Geometry check sheet. Reference: the model listing, model coordinates, mm. Give positions to 0.01 mm unless a question says otherwise; leave off trailing zeros. Loops run counter-clockwise (first coordinate to the right, second up) from the corner with the lowest first, then second, coordinate; pieces in that order, holes last. Notation, with made-up numbers: (-18.5, -0.75) -> (40.5, -0.75) arc R11 cw to (40.5, 7.25) -> close; hole circle Ø2 at (63.5, 82). An arc over 180 degrees is marked (long way). Write item = value, one per line.
```python
from build123d import *

# Parameters (mm, degrees)
F1_DEPTH    = 10.16
F3_D        = 6.35
F4_T1_DEPTH = 76.2


# Not quite as in the source:
# - a fillet or chamfer that OpenCascade refuses, or shapes differently, is made with other operations: its cross-section is extruded or revolved along the edge and cut away or added


with BuildPart() as f1:
    # F0 (on Front) → F1 (new body)
    with BuildSketch(Plane.XZ):
        Polygon((-25.4, 0), (0, 0), (25.4, 0), (25.4, 10.1957246661), (0, 10.1957246661), (-25.4, 10.1957246661), align=None)
    extrude(amount=F1_DEPTH)

    # F3 (through all)
    with Locations(Plane(origin=(0, 0, 0), x_dir=(1, 0, 0), z_dir=(0, 0, -1))):
        with Locations((0.0320593305, 5.0682155415)):
            Hole(F3_D / 2)

    # F4: fillet of radius 5.08 on 4 edges, made by hand

    # F4_s2 → F4_t1 (cut)
    with BuildSketch(Plane.YZ.offset(-38.1)):
        with BuildLine():
            ThreePointArc((-10.16, 5.1157246661), (-8.6721024484, 8.7078271145), (-5.08, 10.1957246661))
            Line((-5.08, 10.1957246661), (-10.16, 10.1957246661))
            Line((-10.16, 10.1957246661), (-10.16, 5.1157246661))
        make_face()
        with BuildLine():
            ThreePointArc((0, 5.1157246661), (-1.4878975516, 8.7078271145), (-5.08, 10.1957246661))
            Line((-5.08, 10.1957246661), (0, 10.1957246661))
            Line((0, 10.1957246661), (0, 5.1157246661))
        make_face()
        with BuildLine():
            ThreePointArc((-5.08, 0), (-8.6721024484, 1.4878975516), (-10.16, 5.08))
            Line((-10.16, 5.08), (-10.16, 0))
            Line((-10.16, 0), (-5.08, 0))
        make_face()
        with BuildLine():
            ThreePointArc((-5.08, 0), (-1.4878975516, 1.4878975516), (0, 5.08))
            Line((0, 5.08), (0, 0))
            Line((0, 0), (-5.08, 0))
        make_face()
    extrude(amount=F4_T1_DEPTH, mode=Mode.SUBTRACT)


solid = f1.part
```
Item 1: Section check A-A, the plane y = -7.75. Record the cut outline in (x, z), plus the area to 3 significant figures.
Answer:
outline = (-25.4, 0.76) -> (-1.67, 0.76) -> (-1.67, 9.44) -> (-25.4, 9.44) -> close; (1.73, 0.76) -> (25.4, 0.76) -> (25.4, 9.44) -> (1.73, 9.44) -> close
area = 411 mm^2
Item 2: Section check B-B, the plane z = 8. Record the cut outline in (x, y) (3 decimals).
Answer:
outline = (-25.4, -9.262) -> (25.4, -9.262) -> (25.4, -0.898) -> (-25.4, -0.898) -> close; hole circle Ø6.35 at (0.032, -5.068)
Item 3: Section check D-D, the plane z = 2. Record the cut outline in (x, y) (3 decimals).
Answer:
outline = (-25.4, -9.12) -> (25.4, -9.12) -> (25.4, -1.04) -> (-25.4, -1.04) -> close; hole circle Ø6.35 at (0.032, -5.068)
Item 4: Draft check along X on faces 1 (the flat face through (-25.4, -5, 5)), 2 (the cylindrical face through (3.204, -5.208, 5.169)), 3 (the flat face through (25.4, -5, 5)). Enter one of: +X half, -X half, draft (parallel to the pull), parting line (faces both ways), or undercut.
Answer:
face_1 = -X half
face_2 = undercut
face_3 = +X half
Item 5: Thickness scan on L1, parallel to X at y = -5.25, z = 1.75; L2, parallel to X at y = -6.5, z = 4.5; L3, parallel to Y at x = 1, z = 5.5. Record the ranges inside material, lowest first. Write a range as [from, to].
Answer:
L1 = [-25.4, -3.14], [3.2, 25.4]
L2 = [-25.4, -2.8], [2.87, 25.4]
L3 = [-10.15, -8.09], [-2.04, -0.01]
Item 6: Gauge pin test, flat ends, axial feed: pin 1 (1 mm diameter, centred on x = -13.5, y = -9, fed in from +Z); pin 2 (1.5 mm diameter, centred on x = 12, y = -7.5, fed in from +Z); pin 3 (2 mm diameter, centred on x = 5, y = -7, fed in from -Z). Record the tip position at first contact, or that the pin passes through.
Answer:
pin_1 = 8.87
pin_2 = 9.91
pin_3 = 0.08
